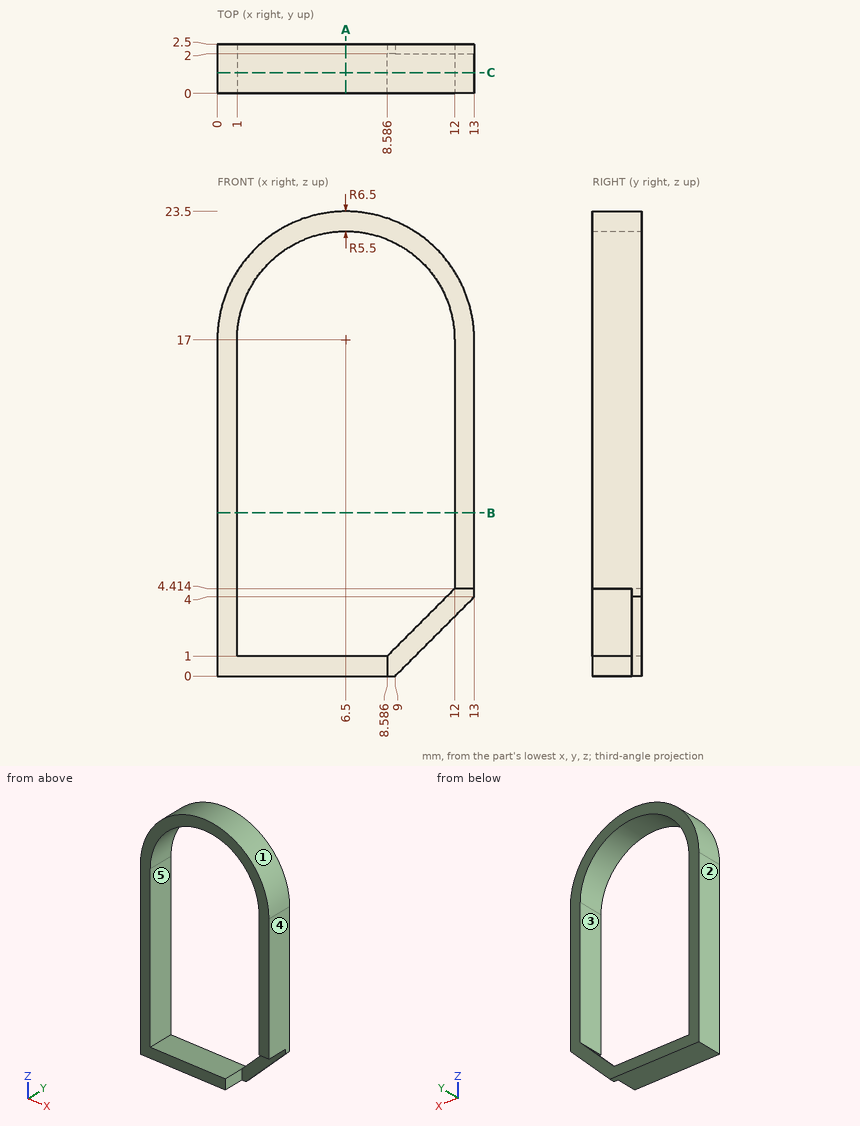
Geometry: see drawing. Coordinates: mm, zero at the bounding-box minimum. A direction names the side the tool comes from. Give positions to 0.01 mm unless a question says otherwise; leave off trailing zeros. Order: outer loops, then holes, each group sorted by start corner. A loop starts at its lowest first (then second) coordinate and runs counter-clockwise, first axis right, second up. Notation, with made-up numbers: M -6.75,37.25 L 22.25,37.25 A12 ccw 22.25,48.25 Z; hole C -11,-12.5 d5. An arc over 180 degrees is marked long. Answer as CSV lines item,"result". Start each with the question number.
1) Cut plane B-B (z = 8.25). Output: boundary loops of the cut face in (x, y).
2) Line query: line 1 (Z direction, x = 6.75, y = 1.15) (1 decimal); line 2 (X direction, y = 0.85, z = 7.75); line 3 (X direction, y = 1.45, z = 1.75). Output: solid intervals per line, ascending. Write a range as from..to.
3) Set-up query: the marked faces 4 and 5. Return all of +Z, -Z, +X, -X, +Y, -Y with unobstructed straight access to the full face (end or side cutting, diameter ignored); none if empty.
4) First-contact query: P1, Ø0.5, axis at y = 1, z = 0.5, coming from the +X side; P2, Ø4, axis at x = 1.5, z = 21, coming from the -Y side; P3, Ø0.5, axis at x = 12.5, y = 1.5, coming from the -Z side. Flat tips, straight axial feed; report the tip coordinate or a pass-through.
5) Cut plane C-C (y = 1.05). Output: boundary loops of the cut face in (x, z).
6) Cut plane A-A (x = 6.5). Output: boundary loops of the cut face in (y, z).
7) Mould query, pull axis X, two halves, no side actions, for the marked faces 1, 2 and 3. Classes: +X half, -X half, draft (parallel to the pull), parting line (faces both ways), or undercut.
Findings below:
1,outline,"M 0,0 L 1,0 L 1,2.5 L 0,2.5 Z; M 12,0 L 13,0 L 13,2.5 L 12,2.5 Z"
2,line 1,"z = 0..1, 22.5..23.5"
2,line 2,"x = 0..1, 12..13"
2,line 3,"x = 0..1"
3,face 4,"+Z, -Z, +X, +Y, -Y"
3,face 5,"+Y, -Y"
4,P1,"stops at x = 8.59"
4,P2,"stops at y = 0"
4,P3,"stops at z = 4.41"
5,outline,"M 0,0 L 8.59,0 L 8.59,1 L 1,1 L 1,17 A5.5 cw 12,17 L 12,4.41 L 13,4.41 L 13,17 A6.5 ccw 0,17 Z"
6,outline,"M 0,0 L 2.5,0 L 2.5,1 L 0,1 Z; M 0,22.5 L 2.5,22.5 L 2.5,23.5 L 0,23.5 Z"
7,face 1,"parting line"
7,face 2,"-X half"
7,face 3,"undercut"
